Check sheet for the modelled part. Datum: model origin and axes. Units: mm. A direction names the side the tool comes from. Round coordinates to 2 decimals unless told otherwise and drop trailing zeros. Loops run counter-clockwise (first coordinate to the right, second up) from the corner with the lowest first, then second, coordinate; pieces in that order, holes last. Notation, with made-up numbers: (89, 83) -> (95, 83) arc R20 cw to (95, 101) -> close; hole circle Ø1 at (-27.75, 18.25). An arc over 180 degrees is marked (long way). One line per item, written item: value. Start each with the question number.
1. Go/stop test with flat-tipped pins: pin 1 (5 mm diameter, centred on x = 130, z = -41, fed in from +Y); pin 2 (1 mm diameter, centred on y = 11, z = -76.5, fed in from -X); pin 3 (2 mm diameter, centred on x = -5, y = 12, fed in from -Z); pin 4 (3 mm diameter, centred on x = 147.5, z = 59.5, fed in from -Y). Record where each tip stops, or that it passes through.
2. Cross-section at A-A on x = 156. Record the cut outline in (y, z), then the cut area to 3 significant figures.
3. Material ranges on L1, parallel to Z at x = 27, y = 14; L2, parallel to Z at x = 52.5, y = 10.75; L3, parallel to Z at x = 58.5, y = 10.25, recorded low to high.
4. Release check for a two-part mould opening along Z. For faces 1 (the face through (-5, 13, 79.288)), 2 (the face through (162, 15, 0)), 3 (the face through (167.14, 13, -38)) record: +Z half, -Z half, draft (parallel to the pull), parting line (faces both ways), or undercut.
5. Set-up check for faces 4 (the face through (-5, 5, 75.588)), 5 (the face through (79, 3, -1)), 6 (the face through (170.04, 7.6, 82.01)), 7 (the face through (62, 12, 77)): record each of +Z, -Z, +X, -X, +Y, -Y from which the full face is reachable in a straight line by a thin tool's end or side.
6. Cross-section at C-C on x = 103. Record the cut outline in (y, z).
7. Cross-section at B-B on z = 65.5. Record the cut outline in (x, y), then the cut area to 3 significant figures.
from build123d import *

# Parameters (mm, degrees)
SKETCH1_W           = 159.54
SKETCH1_H           = 142.875
BOSS_EXTRUDE1_DEPTH = 3
BOSS_EXTRUDE2_DEPTH = 15
CUT_EXTRUDE1_DEPTH  = 3
CUT_EXTRUDE2_DEPTH  = 2
CUT_EXTRUDE3_DEPTH  = 12
CUT_EXTRUDE4_DEPTH  = 12
SKETCH8_R           = 1.1
SKETCH8_R_2         = 1.35
BOSS_EXTRUDE3_DEPTH = 10
BOSS_EXTRUDE5_DEPTH = 10
FILLET3_R           = 5
FILLET4_R           = 5


with BuildPart() as part:
    # Sketch1 → Boss-Extrude1 (new body)
    with BuildSketch(Plane(origin=(0, 0, 0), x_dir=(1, 0, 0), z_dir=(0, 1, 0))):
        with Locations((79.77, 0)):
            Rectangle(SKETCH1_W, SKETCH1_H)
    extrude(amount=BOSS_EXTRUDE1_DEPTH)

    # Sketch3 → Boss-Extrude2 (add)
    with BuildSketch(Plane(origin=(0, 0, 0), x_dir=(1, 0, 0), z_dir=(0, 1, 0))):
        Polygon((0, 71.4375), (0, 83.4375), (171.54, 83.4375), (171.54, -83.4375), (0, -83.4375), (0, -71.4375), (159.54, -71.4375), (159.54, 71.4375), align=None)
    extrude(amount=BOSS_EXTRUDE2_DEPTH)

    # Sketch4 → Cut-Extrude1 (cut)
    with BuildSketch(Plane(origin=(0, 15, 0), x_dir=(1, 0, 0), z_dir=(0, 1, 0))):
        Polygon((46.52, 74.7375), (46.52, 71.4375), (40.22, 71.4375), (40.22, 74.735860656), (15.770004479, 74.735860656), (15.770004479, 78.735860656), (70.969180322, 79.037499922), (70.97, 74.7375), align=None)
        Polygon((121.11, 74.7375), (121.11, 71.4375), (114.81, 71.4375), (114.81, 74.735860656), (90.360004479, 74.735860656), (90.360004479, 78.735860656), (145.559180322, 79.037499922), (145.56, 74.7375), align=None)
        Polygon((145.56, -74.7375), (121.11, -74.7375), (121.11, -71.4375), (114.81, -71.4375), (114.81, -74.735860656), (90.360004479, -74.735860656), (90.360004479, -78.735860656), (145.559180322, -79.037499922), align=None)
        Polygon((70.97, -74.7375), (46.52, -74.7375), (46.52, -71.4375), (40.22, -71.4375), (40.22, -74.735860656), (15.770004479, -74.735860656), (15.770004479, -78.735860656), (70.969180322, -79.037499922), align=None)
        Polygon((159.54, -36.8875), (162.84, -36.8875), (162.84, -16.8875), (167.14, -16.8875), (167.14, -62.8875), (162.84, -62.8875), (162.84, -43.1875), (159.54, -43.1875), align=None)
        Polygon((159.54, 39.8375), (162.84, 39.8375), (162.84, 64.788405135), (167.14, 64.788405135), (167.14, 9.588405135), (162.84, 9.588405135), (162.84, 33.5375), (159.54, 33.5375), align=None)
    extrude(amount=-CUT_EXTRUDE1_DEPTH, mode=Mode.SUBTRACT)

    # Sketch5 → Cut-Extrude2 (cut)
    with BuildSketch(Plane(origin=(0, 12, 0), x_dir=(1, 0, 0), z_dir=(0, 1, 0))):
        Polygon((40.226803468, -71.4375), (40.226803468, -74.7375), (34.114303468, -74.7375), (34.114303468, -78.836104198), (52.639026882, -78.93733368), (52.639026882, -74.7375), (46.525702928, -74.7375), (46.525702928, -71.4375), align=None)
        Polygon((114.817365037, -74.735860656), (108.704865037, -74.735860656), (108.704865037, -78.836107266), (127.229588452, -78.937336748), (127.229588452, -74.735860656), (121.117088452, -74.735860656), (121.117088452, -71.4375), (114.817365037, -71.4375), align=None)
        Polygon((114.817365037, 71.4375), (114.817365037, 74.735860656), (108.704865037, 74.735860656), (108.704865037, 78.836107266), (127.229588452, 78.937336748), (127.229588452, 74.735860656), (121.117088452, 74.735860656), (121.117088452, 71.4375), align=None)
        Polygon((46.525702928, 71.4375), (40.226803468, 71.4375), (40.226803468, 74.7375), (34.114303468, 74.7375), (34.114303468, 78.836104198), (52.639026882, 78.93733368), (52.639026882, 74.7375), (46.525702928, 74.7375), align=None)
        Polygon((162.84, -31.8125), (167.14, -31.8125), (167.14, -48.2625), (162.84, -48.2625), (162.84, -43.1875), (159.54, -43.1875), (159.54, -36.8875), (162.84, -36.8875), align=None)
        Polygon((159.54, 39.8375), (162.84, 39.8375), (162.84, 45.524773716), (167.14, 45.524773716), (167.14, 27.850226284), (162.84, 27.850226284), (162.84, 33.5375), (159.54, 33.5375), align=None)
    extrude(amount=-CUT_EXTRUDE2_DEPTH, mode=Mode.SUBTRACT)

    # Sketch6 → Cut-Extrude3 (cut)
    with BuildSketch(Plane(origin=(171.54, 0, 0), x_dir=(0, 0, -1), z_dir=(1, 0, 0))):
        with BuildLine():
            Line((-11.3875, 10.5), (4.9925, 10.5))
            ThreePointArc((4.9925, 10.5), (7.9925, 7.5), (4.9925, 4.5))
            Line((4.9925, 4.5), (-11.3875, 4.5))
            ThreePointArc((-11.3875, 4.5), (-14.3875, 7.5), (-11.3875, 10.5))
        make_face()
    extrude(amount=-CUT_EXTRUDE3_DEPTH, mode=Mode.SUBTRACT)

    # Sketch7 → Cut-Extrude4 (cut)
    with BuildSketch(Plane(origin=(0, 0, -83.4375), x_dir=(-1, 0, 0), z_dir=(0, 0, -1))):
        with BuildLine():
            Line((-4.24, 10.6343), (12.14, 10.6343))
            ThreePointArc((12.14, 10.6343), (15.14, 7.6343), (12.14, 4.6343))
            Line((12.14, 4.6343), (-4.24, 4.6343))
            ThreePointArc((-4.24, 4.6343), (-7.24, 7.6343), (-4.24, 10.6343))
        make_face()
    extrude(amount=-CUT_EXTRUDE4_DEPTH, mode=Mode.SUBTRACT)

    # Sketch8 → Boss-Extrude3 (add)
    with BuildSketch(Plane.ZY):
        with Locations(Location((-77.4375, 12.81715, 0), (0, 0, 180))):
            Circle(SKETCH8_R)
        with Locations(Location((-77.4375, 2.328843142, 0), (0, 0, 180))):
            Circle(SKETCH8_R_2)
    extrude(amount=BOSS_EXTRUDE3_DEPTH)

    # Sketch9 → Boss-Extrude5 (add)
    with BuildSketch(Plane.ZY):
        Polygon((75.5875, 14.9834354), (79.2875, 14.9834354), (79.2875, 10.85), (83.421238753, 10.85), (83.421238753, 7.15), (79.2875, 7.15), (79.2875, 3.0165646), (75.5875, 3.0165646), (75.5875, 7.15000001), (71.454555518, 7.15000001), (71.454180357, 10.84999999), (75.5875, 10.84999999), align=None)
    extrude(amount=BOSS_EXTRUDE5_DEPTH)

    # Fillet3
    fillet3_edges = [part.edges().sort_by_distance(p)[0] for p in [
        (171.54, 7.5, 83.4375),
    ]]
    fillet(fillet3_edges, radius=FILLET3_R)

    # Fillet4
    fillet4_edges = [part.edges().sort_by_distance(p)[0] for p in [
        (171.54, 7.5, -83.4375),
    ]]
    fillet(fillet4_edges, radius=FILLET4_R)


solid = part.part
Taken from the geometry:
1. pin 1: stops at y = 3
1. pin 2: stops at x = 0
1. pin 3: stops at z = -78.54
1. pin 4: stops at y = 0
2. outline: (0, -83.44) -> (15, -83.44) -> (15, -71.44) -> (3, -71.44) -> (3, 71.44) -> (15, 71.44) -> (15, 83.44) -> (0, 83.44) -> close
2. area: 789 mm2
3. L1: z = -83.44 to -78.8, -74.74 to -71.44, 71.44 to 74.74, 78.8 to 83.44
3. L2: z = -83.44 to -78.94, -74.74 to -71.44, 71.44 to 74.74, 78.94 to 83.44
3. L3: z = -83.44 to -71.44, 71.44 to 83.44
4. face 1: +Z half
4. face 2: draft
4. face 3: undercut
5. face 4: -X, -Y
5. face 5: -X, +Y
5. face 6: +Z, +X, +Y, -Y
5. face 7: +Y
6. outline: (0, -83.44) -> (15, -83.44) -> (15, -78.8) -> (12, -78.8) -> (12, -74.74) -> (15, -74.74) -> (15, -71.44) -> (3, -71.44) -> (3, 71.44) -> (15, 71.44) -> (15, 74.74) -> (12, 74.74) -> (12, 78.8) -> (15, 78.8) -> (15, 83.44) -> (0, 83.44) -> close
7. outline: (0, 0) -> (171.54, 0) -> (171.54, 15) -> (159.54, 15) -> (159.54, 3) -> (0, 3) -> close
7. area: 659 mm2
